Verification items for the finished model (mm, model axes). Coordinates: 2 decimals unless noted, no trailing zeros. Order: outer loops, then holes, each group sorted by start corner. A loop starts at its lowest first (then second) coordinate and runs counter-clockwise, first axis right, second up. Notation, with made-up numbers: M 76,63 L 89,63 A34 ccw 89,97 Z; hole C -38.5,-21.5 d9. An arc over 180 degrees is marked long. Return JSON: item names as keys, results as strings.
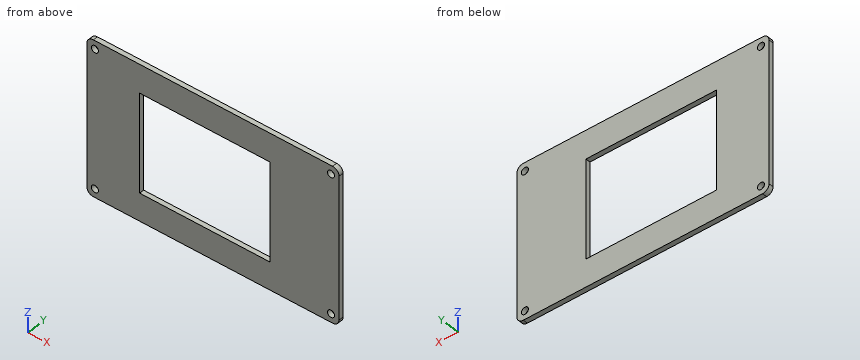
```python
from build123d import *

# Parameters (mm, degrees)
SKETCH1_W           = 78.86
SKETCH1_H           = 48
SKETCH1_W_2         = 40.8
SKETCH1_H_2         = 30.6
BOSS_EXTRUDE1_DEPTH = 1.5
CUT_EXTRUDE1_REACH  = 48.184
SKETCH2_R           = 1.1
FILLET1_R           = 2


with BuildPart() as part:
    # Sketch1 → Boss-Extrude1 (new body)
    with BuildSketch(Plane(origin=(0, 0, 0), x_dir=(1, 0, 0), z_dir=(0, 1, 0))):
        Rectangle(SKETCH1_W, SKETCH1_H)
        with Locations((-2.54, 0.12)):
            Rectangle(SKETCH1_W_2, SKETCH1_H_2, mode=Mode.SUBTRACT)
    extrude(amount=BOSS_EXTRUDE1_DEPTH)

    # Sketch2 → Cut-Extrude1 (cut, up to next)
    with BuildSketch(Plane(origin=(0, 1.5, 0), x_dir=(1, 0, 0), z_dir=(0, 1, 0)), mode=Mode.PRIVATE) as cut_extrude1_sk1:
        with Locations(Location((-36.93, 21.375, 0), (0, 0, 270))):
            Circle(SKETCH2_R)
    cut_extrude1_tool1 = extrude(cut_extrude1_sk1.sketch, amount=-CUT_EXTRUDE1_REACH, mode=Mode.PRIVATE) & part.part
    # Sketch2 → Cut-Extrude1 (cut, up to next)
    with BuildSketch(Plane(origin=(0, 1.5, 0), x_dir=(1, 0, 0), z_dir=(0, 1, 0)), mode=Mode.PRIVATE) as cut_extrude1_sk2:
        with Locations(Location((-36.93, -21.375, 0), (0, 0, 270))):
            Circle(SKETCH2_R)
    cut_extrude1_tool2 = extrude(cut_extrude1_sk2.sketch, amount=-CUT_EXTRUDE1_REACH, mode=Mode.PRIVATE) & part.part
    # Sketch2 → Cut-Extrude1 (cut, up to next)
    with BuildSketch(Plane(origin=(0, 1.5, 0), x_dir=(1, 0, 0), z_dir=(0, 1, 0)), mode=Mode.PRIVATE) as cut_extrude1_sk3:
        with Locations(Location((36.93, 21.375, 0), (0, 0, 270))):
            Circle(SKETCH2_R)
    cut_extrude1_tool3 = extrude(cut_extrude1_sk3.sketch, amount=-CUT_EXTRUDE1_REACH, mode=Mode.PRIVATE) & part.part
    # Sketch2 → Cut-Extrude1 (cut, up to next)
    with BuildSketch(Plane(origin=(0, 1.5, 0), x_dir=(1, 0, 0), z_dir=(0, 1, 0)), mode=Mode.PRIVATE) as cut_extrude1_sk4:
        with Locations(Location((36.93, -21.375, 0), (0, 0, 270))):
            Circle(SKETCH2_R)
    cut_extrude1_tool4 = extrude(cut_extrude1_sk4.sketch, amount=-CUT_EXTRUDE1_REACH, mode=Mode.PRIVATE) & part.part
    add(cut_extrude1_tool1.solids().sort_by_distance((-36.93, 1.5, -21.375))[0], mode=Mode.SUBTRACT)
    add(cut_extrude1_tool2.solids().sort_by_distance((-36.93, 1.5, 21.375))[0], mode=Mode.SUBTRACT)
    add(cut_extrude1_tool3.solids().sort_by_distance((36.93, 1.5, -21.375))[0], mode=Mode.SUBTRACT)
    add(cut_extrude1_tool4.solids().sort_by_distance((36.93, 1.5, 21.375))[0], mode=Mode.SUBTRACT)

    # Fillet1
    fillet1_edges = [part.edges().sort_by_distance(p)[0] for p in [
        (-39.43, 0.75, -24),
        (39.43, 0.75, -24),
        (39.43, 0.75, 24),
        (-39.43, 0.75, 24),
    ]]
    fillet(fillet1_edges, radius=FILLET1_R)


solid = part.part
```
Q1. Go/stop test with a flat-tipped pin: pin 1 (1.8 mm diameter, centred on x = -36.93, z = -21.375, fed in from +Y). Record where the tip stops, or that it passes through.
Values:
{"pin 1": "through"}
Q2. Cross-section at C-C, the plane y = 0.7. Record the boundary of the cut face in (x, z) (3 decimals).
Values:
{"outline": "M -39.43,-22 A2 ccw -37.43,-24 L 37.43,-24 A2 ccw 39.43,-22 L 39.43,22 A2 ccw 37.43,24 L -37.43,24 A2 ccw -39.43,22 Z; hole C -36.93,-21.375 d2.2; hole C -36.93,21.375 d2.2; hole M -22.94,-15.42 L 17.86,-15.42 L 17.86,15.18 L -22.94,15.18 Z; hole C 36.93,-21.375 d2.2; hole C 36.93,21.375 d2.2"}
Q3. Cross-section at B-B, the plane z = -7.5. Record the boundary of the cut face in (x, y).
Values:
{"outline": "M -39.43,0 L -22.94,0 L -22.94,1.5 L -39.43,1.5 Z; M 17.86,0 L 39.43,0 L 39.43,1.5 L 17.86,1.5 Z"}
Q4. Cross-section at A-A, the plane x = -20.5. Record the boundary of the cut face in (y, z), and give its area (3 significant figures).
Values:
{"outline": "M 0,-24 L 1.5,-24 L 1.5,-15.42 L 0,-15.42 Z; M 0,15.18 L 1.5,15.18 L 1.5,24 L 0,24 Z", "area": "26.1 mm^2"}
Q5. Material ranges on line 1 along X through (y, z) = (0.1, -8.5); line 2 along X through (y, z) = (0.8, -21.5); line 3 along Z through (x, y) = (-11, 0.45), recorded low to high.
Values:
{"line 1": "-39.43 to -22.94, 17.86 to 39.43", "line 2": "-39.43 to -38.02, -35.84 to 35.84, 38.02 to 39.43", "line 3": "-24 to -15.42, 15.18 to 24"}
